Here's how the part is built. I have some questions about the finished solid (model axes, mm). A direction names the side the tool comes from. Round coordinates to 2 decimals unless told otherwise and drop trailing zeros. Loops run counter-clockwise (first coordinate to the right, second up) from the corner with the lowest first, then second, coordinate; pieces in that order, holes last. Notation, with made-up numbers: M 50.5,-7.75 L 89.5,-7.75 A12 ccw 89.5,1.25 Z; hole C 6,56 d3. An arc over 180 degrees is marked long. Use a Markdown table: item, result.
```python
from build123d import *

# Parameters (mm, degrees)
F0_W      = 101.6
F0_H      = 7.62
F1_DEPTH  = 7.62
F2_W      = 5.08
F2_H      = 7.62
F3_DEPTH  = 7.62
F4_R      = 2.54
F5_DEPTH  = 25.4
F6_W      = 22.86
F6_H      = 22.86
F6_W_2    = 7.62
F6_H_2    = 7.62
F7_DEPTH  = 50.8
F8_R      = 6.35
F8_R_2    = 3.81
F9_DEPTH  = 50.8
F10_W     = 50.8
F10_H     = 2.54
F11_DEPTH = 12.7
F12_W     = 2.54
F12_H     = 6.35
F12_W_2   = 15.24
F13_DEPTH = 6.35
F14_W     = 2.54
F14_H     = 6.35
F14_W_2   = 15.24
F15_DEPTH = 6.35
F16_R     = 1.27
F17_DEPTH = 25.4
F18_R     = 1.27
F19_DEPTH = 25.4


with BuildPart() as f1:
    # F0 (on Right) → F1 (new body)
    with BuildSketch(Plane.YZ):
        with Locations((-1.6321643911, 33.6084578316)):
            Rectangle(F0_W, F0_H)
    extrude(amount=F1_DEPTH)

    # F2 (on face) → F3 (join)
    with BuildSketch(Plane.XZ.offset(52.4321643911)):
        with Locations((3.81, 33.6084578316)):
            Rectangle(F2_W, F2_H)
    extrude(amount=F3_DEPTH)

    # F4 (on face) → F5 (cut)
    with BuildSketch(Plane.YZ.offset(6.35)):
        with Locations((-56.2421643911, 33.6084578316)):
            Circle(F4_R)
        with BuildLine():
            ThreePointArc((-56.2421643911, 29.7984578316), (-59.9211503168, 33.6084578316), (-56.2421643911, 37.4184578316))
            Line((-56.2421643911, 37.4184578316), (-60.0521643911, 37.4184578316))
            Line((-60.0521643911, 37.4184578316), (-60.0521643911, 29.7984578316))
            Line((-60.0521643911, 29.7984578316), (-56.2421643911, 29.7984578316))
        make_face()
    extrude(amount=-F5_DEPTH, mode=Mode.SUBTRACT)

    # F6 (on face) → F7 (join)
    with BuildSketch(Plane(origin=(0, 49.1678356089, 0), x_dir=(-1, 0, 0), z_dir=(0, 1, 0))):
        with Locations((-3.81, 33.6136929691)):
            Rectangle(F6_W, F6_H)
        with Locations((-3.81, 33.6084578316)):
            Rectangle(F6_W_2, F6_H_2, mode=Mode.SUBTRACT)
        with Locations((-3.81, 33.6084578316)):
            Rectangle(F6_W_2, F6_H_2)
    extrude(amount=F7_DEPTH)

    # F8 (on face) → F9 (join)
    with BuildSketch(Plane(origin=(0, 99.9678356089, 0), x_dir=(-1, 0, 0), z_dir=(0, 1, 0))):
        with Locations((-3.81, 33.6136929691)):
            Circle(F8_R)
        with Locations((-3.81, 33.6136929691)):
            Circle(F8_R_2, mode=Mode.SUBTRACT)
    extrude(amount=F9_DEPTH)

    # F10 (on face) → F11 (join)
    with BuildSketch(Plane.YZ.offset(15.24)):
        with Locations((74.5678356089, 33.6136929691)):
            Rectangle(F10_W, F10_H)
    extrude(amount=F11_DEPTH)

    # F12 (on face) → F13 (join)
    with BuildSketch(Plane.YZ.offset(15.24)):
        with Locations((63.1378356089, 38.0586929691)):
            Rectangle(F12_W, F12_H)
        with Locations((74.5678356089, 38.0586929691)):
            Rectangle(F12_W_2, F12_H)
        with Locations((85.9978356089, 38.0586929691)):
            Rectangle(F12_W, F12_H)
    extrude(amount=F13_DEPTH)

    # F14 (on face) → F15 (join)
    with BuildSketch(Plane.YZ.offset(15.24)):
        with Locations((63.1378356089, 29.1686929691)):
            Rectangle(F14_W, F14_H)
        with Locations((74.5678356089, 29.1686929691)):
            Rectangle(F14_W_2, F14_H)
        with Locations((85.9978356089, 29.1686929691)):
            Rectangle(F14_W, F14_H)
    extrude(amount=F15_DEPTH)

    # F16 (on face) → F17 (cut)
    with BuildSketch(Plane.XZ.offset(-61.8678356089)):
        with Locations((18.415, 38.0586929691)):
            Circle(F16_R)
    extrude(amount=-F17_DEPTH, mode=Mode.SUBTRACT)

    # F18 (on face) → F19 (cut)
    with BuildSketch(Plane.XZ.offset(-61.8678356089)):
        with Locations((18.415, 29.1686929691)):
            Circle(F18_R)
    extrude(amount=-F19_DEPTH, mode=Mode.SUBTRACT)


solid = f1.part
```
Q1. I need wall thicknesses on line 1 (Y direction, x = 18.5, z = 40.5); line 2 (Z direction, x = 3.81, y = 117); line 3 (X direction, y = 141, z = 34). Which ranges of each line are inside material? Lowest first, please. Write a range as from..to.
Return value:
| item | result |
|---|---|
| line 1 | y = 61.87..64.41, 66.95..82.19, 84.73..87.27 |
| line 2 | z = 27.26..29.8, 37.42..39.96 |
| line 3 | x = -2.53..0.02, 7.6..10.15 |
Q2. Imagine slicing it at C-C, the plane z = 24.25. Please give me the cut outline in (x, y).
Return value:
| item | result |
|---|---|
| outline | M -7.62,49.17 L 15.24,49.17 L 15.24,99.97 L -7.62,99.97 Z |
Q3. We'd pull the mould along Z, two halves only. Please class faces 6 (the flat face through (18, 74, 41.234)), 7 (the cylindrical face through (4.636, 125.012, 29.894)), 8 (the flat face through (10.4, 99.968, 33.8)): pulls with the +Z half, pulls with the -Z half, needs draft (parallel to the pull), parting line crosses it, or undercut.
Return value:
| item | result |
|---|---|
| face 6 | pulls with the +Z half |
| face 7 | undercut |
| face 8 | needs draft |
Q4. Imagine slicing it at A-A, the plane x = 3.81. Please give me the cut outline in (y, z).
Return value:
| item | result |
|---|---|
| outline | M -56.24,29.8 L 49.17,29.8 L 49.17,22.18 L 99.97,22.18 L 99.97,27.26 L 150.77,27.26 L 150.77,29.8 L 99.97,29.8 L 99.97,37.42 L 150.77,37.42 L 150.77,39.96 L 99.97,39.96 L 99.97,45.04 L 49.17,45.04 L 49.17,37.42 L -56.24,37.42 A3.81 ccw Z; hole C -56.24,33.61 d5.08 |
Q5. Will these pins go through, and if not, where does the flat tip stop? P1, Ø3, axis at x = 19.5, z = 30.5, coming from the -Y side; P2, Ø6.5, axis at y = -56.24, z = 33.61, coming from the +X side; P3, Ø3, axis at x = 18.5, y = 73.5, coming from the -Z side.
Return value:
| item | result |
|---|---|
| P1 | stops at y = 61.87 |
| P2 | stops at x = 6.35 |
| P3 | stops at z = 25.99 |
Q6. For faces 1 (the flat face through (18.4, 64.408, 36.6)), 2 (the flat face through (18, 64.408, 31)), 3 (the flat face through (1.27, -53.6, 34.4)), 4 (the flat face through (21.59, 74, 38)), 5 (the flat face through (4, -4, 37.418)), which set-ups out of +Z, -Z, +X, -X, +Y, -Y let a thin tool reach every point of the face, with its end or its side?
Return value:
| item | result |
|---|---|
| face 1 | +Z, +X |
| face 2 | -Z, +X |
| face 3 | +Z, -Z, -X, -Y |
| face 4 | +Z, +X, +Y, -Y |
| face 5 | +Z, +X, -X, -Y |
Q7. Imagine slicing it at B-B, the plane y = 23. Please give me the cut outline in (x, z).
Return value:
| item | result |
|---|---|
| outline | M 0,29.8 L 7.62,29.8 L 7.62,37.42 L 0,37.42 Z |
Q8. Imagine slicing it at D-D, the plane y = 137. Please give me the cut outline in (x, z).
Return value:
| item | result |
|---|---|
| outline | C 3.81,33.61 d12.7; hole C 3.81,33.61 d7.62 |
